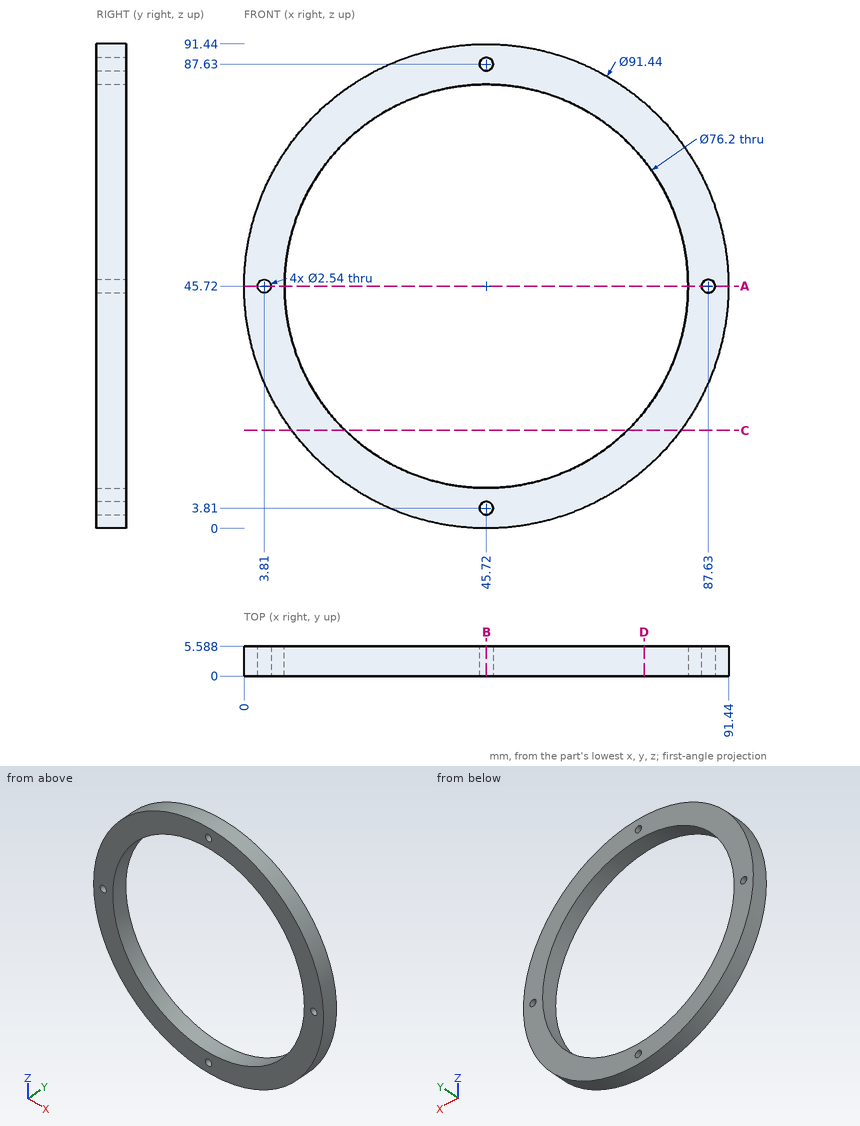
Here's the drawing with two shaded views (mm, measured from the low corner). I have some questions. Give positions to 0.01 mm unless a question says otherwise; leave off trailing zeros. Loops run counter-clockwise (first coordinate to the right, second up) from the corner with the lowest first, then second, coordinate; pieces in that order, holes last. Notation, with made-up numbers: (-38, 12.25) -> (0, 12.25) arc R8 ccw to (0, 20.25) -> close; hole circle Ø6 at (18.25, -5.5). An arc over 180 degrees is marked (long way). Use one line per item in the form item = value.
1) If we section it at D-D (x = 75.5): Please give me the cut outline in (y, z).
Answers:
outline = (0, 11.03) -> (5.59, 11.03) -> (5.59, 21.96) -> (0, 21.96) -> close; (0, 69.48) -> (5.59, 69.48) -> (5.59, 80.41) -> (0, 80.41) -> close
2) If we section it at C-C (z = 18.5): Please give me the cut outline in (x, y).
Answers:
outline = (8.99, 0) -> (19.06, 0) -> (19.06, 5.59) -> (8.99, 5.59) -> close; (72.38, 0) -> (82.45, 0) -> (82.45, 5.59) -> (72.38, 5.59) -> close
3) Will these pins go through, and if not, where does the flat tip stop? pin 1 (2 mm diameter, centred on x = 26, y = 4, fed in from -Z); pin 2 (1.5 mm diameter, centred on x = 45.72, z = 3.81, fed in from +Y); pin 3 (1.5 mm diameter, centred on y = 1, z = 22, fed in from +X).
Answers:
pin_1 = 4.01
pin_2 = through
pin_3 = 85.25
4) If we section it at B-B (x = 45.72): Please give me the cut outline in (y, z).
Answers:
outline = (0, 0) -> (5.59, 0) -> (5.59, 2.54) -> (0, 2.54) -> close; (0, 5.08) -> (5.59, 5.08) -> (5.59, 7.62) -> (0, 7.62) -> close; (0, 83.82) -> (5.59, 83.82) -> (5.59, 86.36) -> (0, 86.36) -> close; (0, 88.9) -> (5.59, 88.9) -> (5.59, 91.44) -> (0, 91.44) -> close
5) I need wall thicknesses on line 1 along X through (y, z) = (0.2, 46); line 2 along X through (y, z) = (2.35, 63); line 3 along X through (y, z) = (1.15, 18). Which ranges of each line are inside material? Lowest first, please.
Answers:
line_1 = 0 to 2.57, 5.05 to 7.62, 83.82 to 86.39, 88.87 to 91.44
line_2 = 3.39 to 11.76, 79.68 to 88.05
line_3 = 9.36 to 19.58, 71.86 to 82.08
6) If we section it at A-A (z = 45.72): Please give me the cut outline in (x, y).
Answers:
outline = (0, 0) -> (2.54, 0) -> (2.54, 5.59) -> (0, 5.59) -> close; (5.08, 0) -> (7.62, 0) -> (7.62, 5.59) -> (5.08, 5.59) -> close; (83.82, 0) -> (86.36, 0) -> (86.36, 5.59) -> (83.82, 5.59) -> close; (88.9, 0) -> (91.44, 0) -> (91.44, 5.59) -> (88.9, 5.59) -> close
